For this review, use the dimensioned drawing (mm, ordinates from the lowest corner) and the shaded views. A direction names the side the tool comes from. Coordinates: 2 decimals unless noted, no trailing zeros. Loops run counter-clockwise (first coordinate to the right, second up) from the corner with the lowest first, then second, coordinate; pieces in that order, holes last. Notation, with made-up numbers: (19.5, 82.25) - (50.5, 82.25) arc R14 ccw to (50.5, 108.25) - close; hole circle Ø11 at (65.25, -9). An arc over 180 degrees is marked (long way). Answer in a Markdown table with one row per item. Add a question column.
(1) We need section D-D on x = 11. Write out the cut boundary in (y, z), plus the area to 3 significant figures.
(2) Machinability: for the marked faces 5, 6, 7 and 8, which of the approach directions +Z, -Z, +X, -X, +Y, -Y give a long, thin tool a straight path to every point of the face, cutting with its end or side? Answer none if there is none.
(3) For line 1 along Z through (x, y) = (16.5, 18); line 2 along Y through (x, z) = (15, 42); line 3 along X through (y, z) = (38, 18), list the stretches that pass through material, from the lowest coordinate up.
(4) For P1, Ø5, axis at x = 18, y = 12.5, coming from the -Z side; P2, Ø12, axis at x = 4.5, y = 11, coming from the -Z side; P3, Ø1.5, axis at y = 5, z = 38.5, coming from the -X side; P4, Ø7.5, axis at x = 11.5, z = 2, coming from the +Y side, all flat-tipped, find the tip position at first contact; note any pin that passes through.
(5) We need section A-A on z = 43. Write out the cut boundary in (x, y), plus the area to 3 significant figures.
(6) We need section C-C on x = 6. Write out the cut boundary in (y, z).
(7) Mouldability with a two-part tool opening along Y and no side actions: class the marked faces 1, 2, 3 and 4 as +Y half, -Y half, draft (parallel to the pull), parting line (faces both ways), or undercut.
(8) We need section B-B on y = 23. Write out the cut boundary in (x, z), plus the area to 3 significant figures.
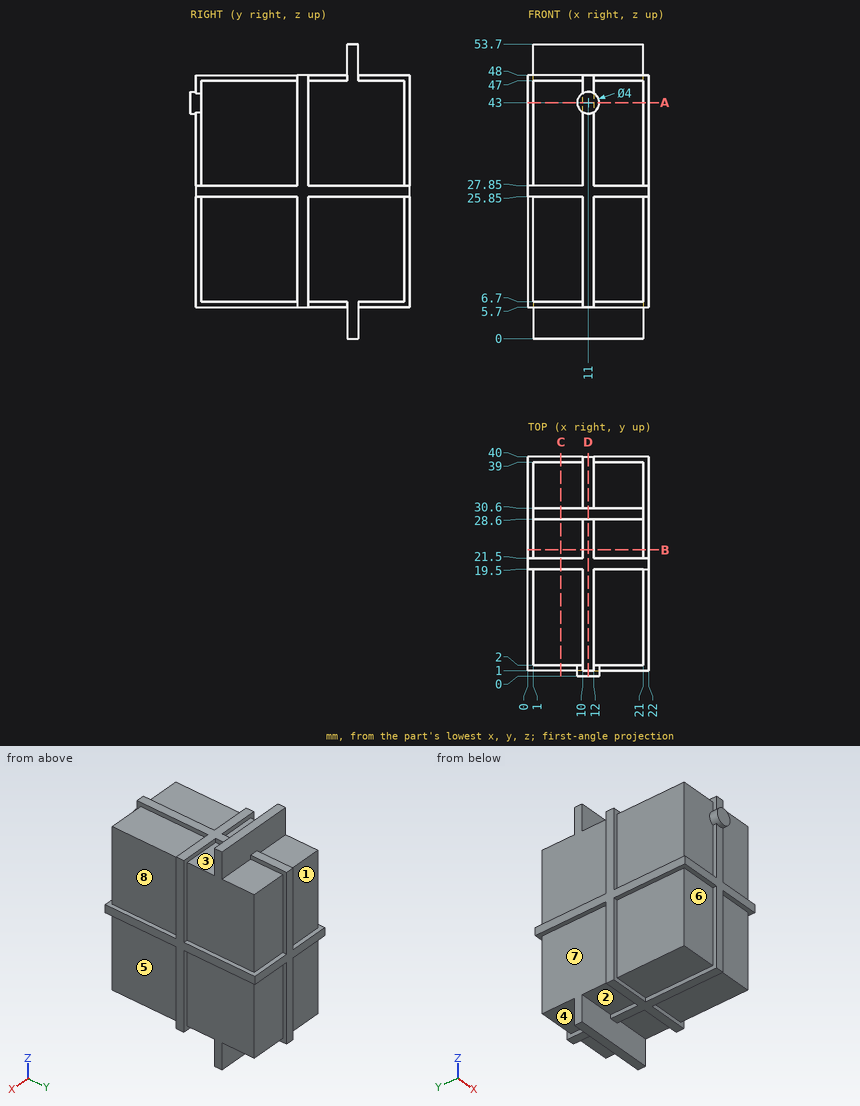
Outcome:
| question | item | result |
|---|---|---|
| 1 | outline | (0, 41) - (1, 41) - (1, 5.7) - (28.6, 5.7) - (28.6, 0) - (30.6, 0) - (30.6, 5.7) - (40, 5.7) - (40, 48) - (30.6, 48) - (30.6, 53.7) - (28.6, 53.7) - (28.6, 48) - (1, 48) - (1, 45) - (0, 45) - close |
| 1 | area | 1,680 mm² |
| 2 | face 5 | -Z, +X, -Y |
| 2 | face 6 | -Z, -X, -Y |
| 2 | face 7 | -Z, -X, +Y |
| 2 | face 8 | +Z, +X, -Y |
| 3 | line 1 | 6.7 to 47 |
| 3 | line 2 | 2 to 39 |
| 3 | line 3 | 1 to 21 |
| 4 | P1 | z = 6.7 |
| 4 | P2 | z = 5.7 |
| 4 | P3 | x = 1 |
| 4 | P4 | y = 40 |
| 5 | outline | (0, 19.5) - (1, 19.5) - (1, 2) - (9, 2) - (9, 0) - (13, 0) - (13, 2) - (21, 2) - (21, 19.5) - (22, 19.5) - (22, 21.5) - (21, 21.5) - (21, 39) - (12, 39) - (12, 40) - (10, 40) - (10, 39) - (1, 39) - (1, 21.5) - (0, 21.5) - close |
| 5 | area | 754 mm² |
| 6 | outline | (1, 25.85) - (2, 25.85) - (2, 6.7) - (19.5, 6.7) - (19.5, 5.7) - (21.5, 5.7) - (21.5, 6.7) - (28.6, 6.7) - (28.6, 0) - (30.6, 0) - (30.6, 6.7) - (39, 6.7) - (39, 25.85) - (40, 25.85) - (40, 27.85) - (39, 27.85) - (39, 47) - (30.6, 47) - (30.6, 53.7) - (28.6, 53.7) - (28.6, 47) - (21.5, 47) - (21.5, 48) - (19.5, 48) - (19.5, 47) - (2, 47) - (2, 27.85) - (1, 27.85) - close |
| 7 | face 1 | +Y half |
| 7 | face 2 | undercut |
| 7 | face 3 | undercut |
| 7 | face 4 | draft |
| 8 | outline | (0, 25.85) - (1, 25.85) - (1, 6.7) - (10, 6.7) - (10, 5.7) - (12, 5.7) - (12, 6.7) - (21, 6.7) - (21, 25.85) - (22, 25.85) - (22, 27.85) - (21, 27.85) - (21, 47) - (12, 47) - (12, 48) - (10, 48) - (10, 47) - (1, 47) - (1, 27.85) - (0, 27.85) - close |
| 8 | area | 814 mm² |
